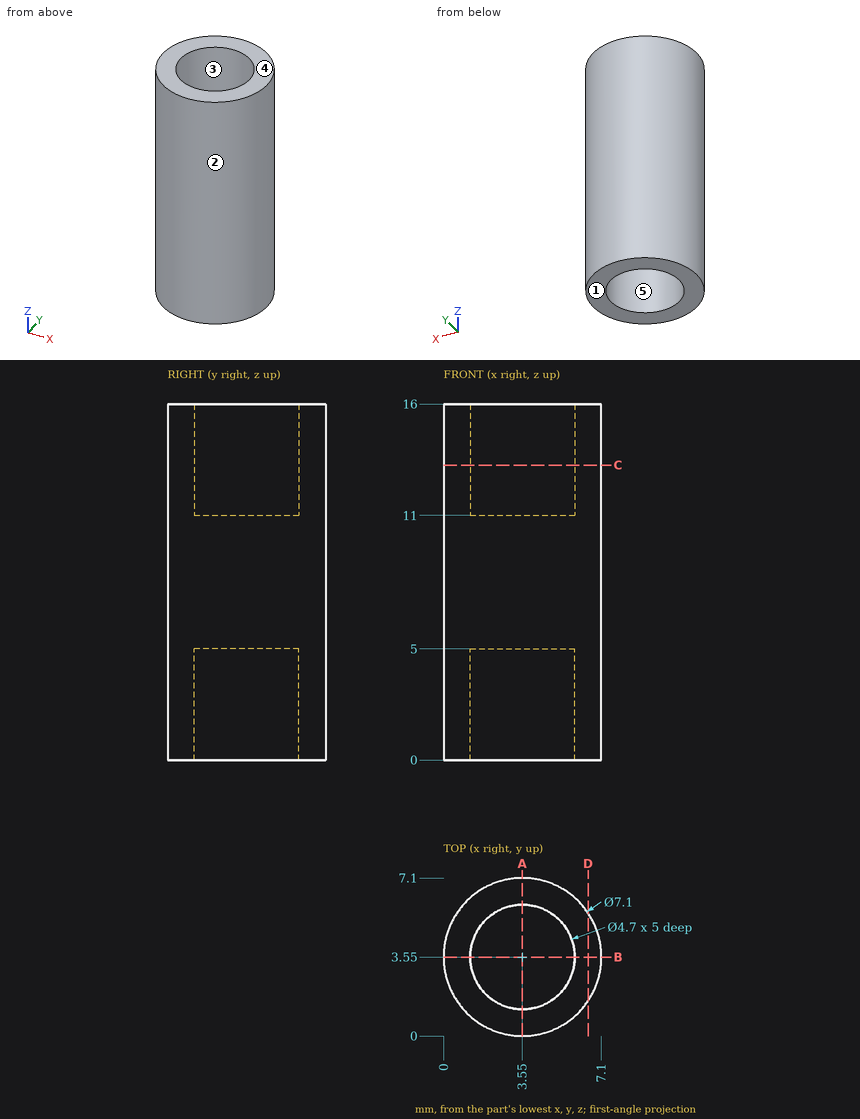
Study the drawing (mm; zero at the part's minimum x, y, z) and answer. A direction names the side the tool comes from. Coordinates: 2 decimals unless noted, no trailing zeros. Write each loop counter-clockwise with the first axis right and the second up, starting at its lowest first coordinate (ties: lowest second). Pieces come first, ordered by that corner, then holes. Notation, with made-up numbers: (8, -24.75) - (67, -24.75) arc R23 cw to (67, 1.25) - close; hole circle Ø1 at (58, 41). An arc over 180 degrees is marked (long way). One line per item, written item: value.
1) Find section C-C (z = 13.25). Give the vertices of the cut face in (x, y).
Geometry check:
outline: circle Ø7.1 at (3.55, 3.55); hole circle Ø4.7 at (3.55, 3.55)
2) Find section A-A (x = 3.55). Give the vertices of the cut face in (y, z), and give its area (3 significant figures).
Geometry check:
outline: (0, 0) - (1.2, 0) - (1.2, 5) - (5.9, 5) - (5.9, 0) - (7.1, 0) - (7.1, 16) - (5.9, 16) - (5.9, 11) - (1.2, 11) - (1.2, 16) - (0, 16) - close
area: 66.6 mm2
3) Each of these flat-tipped pins is pushed along its axis until it touches: pin 1 Ø4 at (x, z) = (6.5, 7.5) entering from -Y; pin 2 Ø1.4 at (x, y) = (4, 3.5) entering from -Z; pin 3 Ø2 at (x, z) = (2, 10.5) entering from -Y. Where does it stop, or does it pass through?
Geometry check:
pin 1: stops at y = 0.13
pin 2: stops at z = 5
pin 3: stops at y = 0.04
4) For a pull along X with two mould halves and no side action, classify the marked faces 1, 2 and 3 as pulls with the +X half, pulls with the -X half, needs draft (parallel to the pull), parting line crosses it, or undercut.
Geometry check:
face 1: needs draft
face 2: parting line crosses it
face 3: undercut
5) Find section D-D (x = 6.5). Give the vertices of the cut face in (y, z), and give its area (3 significant figures).
Geometry check:
outline: (1.58, 0) - (5.52, 0) - (5.52, 16) - (1.58, 16) - close
area: 63.2 mm2
6) Consider line 1 along Y through (x, z) = (3.55, 14.1); line 2 along X through (y, z) = (5.25, 4.5); line 3 along Z through (x, y) = (4.5, 4). Determine where each line is inside the solid, lowest interval first. Write a range as from..to.
Geometry check:
line 1: y = 0..1.2, 5.9..7.1
line 2: x = 0.43..1.93, 5.17..6.67
line 3: z = 5..11
7) A tool of negligible diameter and unlimited length cuts with its end or side. For the marked faces 4 and 5, from which of +Z, -Z, +X, -X, +Y, -Y can it reach the whole face along a straight path? Write none if from no direction.
Geometry check:
face 4: +Z, +X, -X, +Y, -Y
face 5: -Z
